Geometry: see drawing. Coordinates: mm, zero at the bounding-box minimum. Coordinates: 2 decimals unless noted, no trailing zeros. Loops run counter-clockwise (first coordinate to the right, second up) from the corner with the lowest first, then second, coordinate; pieces in that order, holes last. Notation, with made-up numbers: M -38,72.25 L -4,72.25 A24 cw -4,86.25 Z; hole C -28.75,-38.75 d9. An arc over 180 degrees is marked long. Write each question's results on one line, items separated by ' | '. Start each with the question number.
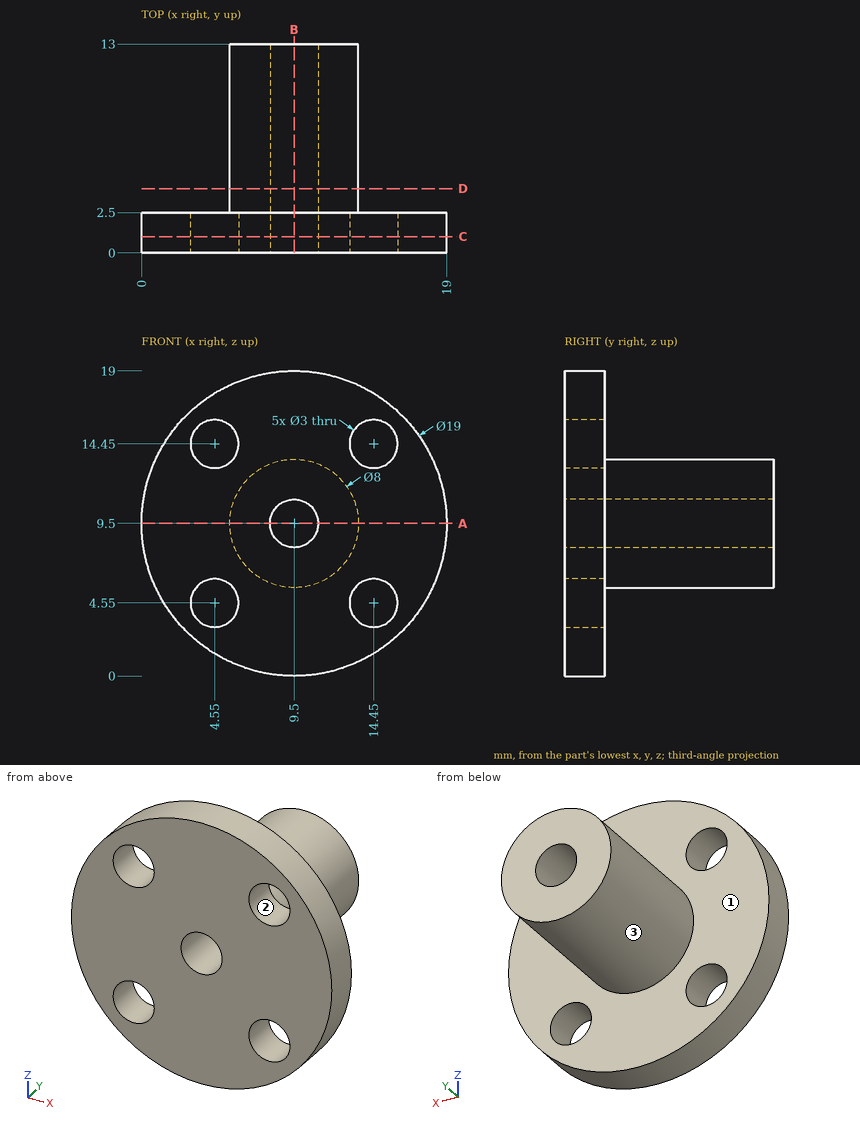
Item 1: Mould query, pull axis Z, two halves, no side actions, for the marked faces 1, 2 and 3. Classes: +Z half, -Z half, draft (parallel to the pull), parting line (faces both ways), or undercut.
Item 2: Cut plane A-A (z = 9.5). Output: boundary loops of the cut face in (x, y), then the cut area to 3 significant figures.
Item 3: Cut plane D-D (y = 4). Output: boundary loops of the cut face in (x, z), then the cut area to 3 significant figures.
Item 4: First-contact query: pin 1 Ø3 at (x, y) = (3, 11) entering from -Z; pin 2 Ø3.5 at (x, z) = (4.55, 14.45) entering from +Y; pin 3 Ø4 at (y, z) = (1.5, 12) entering from +X. Flat tips, straight axial feed; report the tip coordinate or a pass-through.
Item 5: Cut plane B-B (x = 9.5). Output: boundary loops of the cut face in (y, z).
Item 6: Line query: probe 1 along Y at (x, z) = (5.25, 13); probe 2 along Z at (x, y) = (8.75, 11); probe 3 along Z at (x, y) = (10.75, 4.5). Output: solid intervals per line, ascending.
Item 7: Cut plane C-C (y = 1). Output: boundary loops of the cut face in (x, z), then the cut area to 3 significant figures.
Response values:
1) face 1: draft | face 2: undercut | face 3: parting line
2) outline: M 0,0 L 8,0 L 8,13 L 5.5,13 L 5.5,2.5 L 0,2.5 Z; M 11,0 L 19,0 L 19,2.5 L 13.5,2.5 L 13.5,13 L 11,13 Z | area: 92.5 mm2
3) outline: C 9.5,9.5 d8; hole C 9.5,9.5 d3 | area: 43.2 mm2
4) pin 1: passes through | pin 2: stops at y = 2.5 | pin 3: stops at x = 18.99
5) outline: M 0,0 L 2.5,0 L 2.5,5.5 L 13,5.5 L 13,8 L 0,8 Z; M 0,11 L 13,11 L 13,13.5 L 2.5,13.5 L 2.5,19 L 0,19 Z
6) probe 1: y = 0 to 2.5 | probe 2: z = 5.57 to 8.2, 10.8 to 13.43 | probe 3: z = 5.7 to 8.67, 10.33 to 13.3
7) outline: C 9.5,9.5 d19; hole C 4.55,4.55 d3; hole C 4.55,14.45 d3; hole C 9.5,9.5 d3; hole C 14.45,4.55 d3; hole C 14.45,14.45 d3 | area: 248 mm2
